Check sheet for the drawn part. Datum: minimum x, y, z corner. Units: mm. A direction names the side the tool comes from. Round coordinates to 2 decimals unless told otherwise and drop trailing zeros. Write each loop counter-clockwise with the first axis right and the second up, starting at its lowest first coordinate (ties: lowest second). Pieces come first, ordered by that corner, then holes. Notation, with made-up numbers: M 11,69.5 L 39,69.5 A17 ccw 39,97.5 Z; hole C 47,35 d11. An arc over 180 degrees is marked long. Put each result on its own line as item: value.
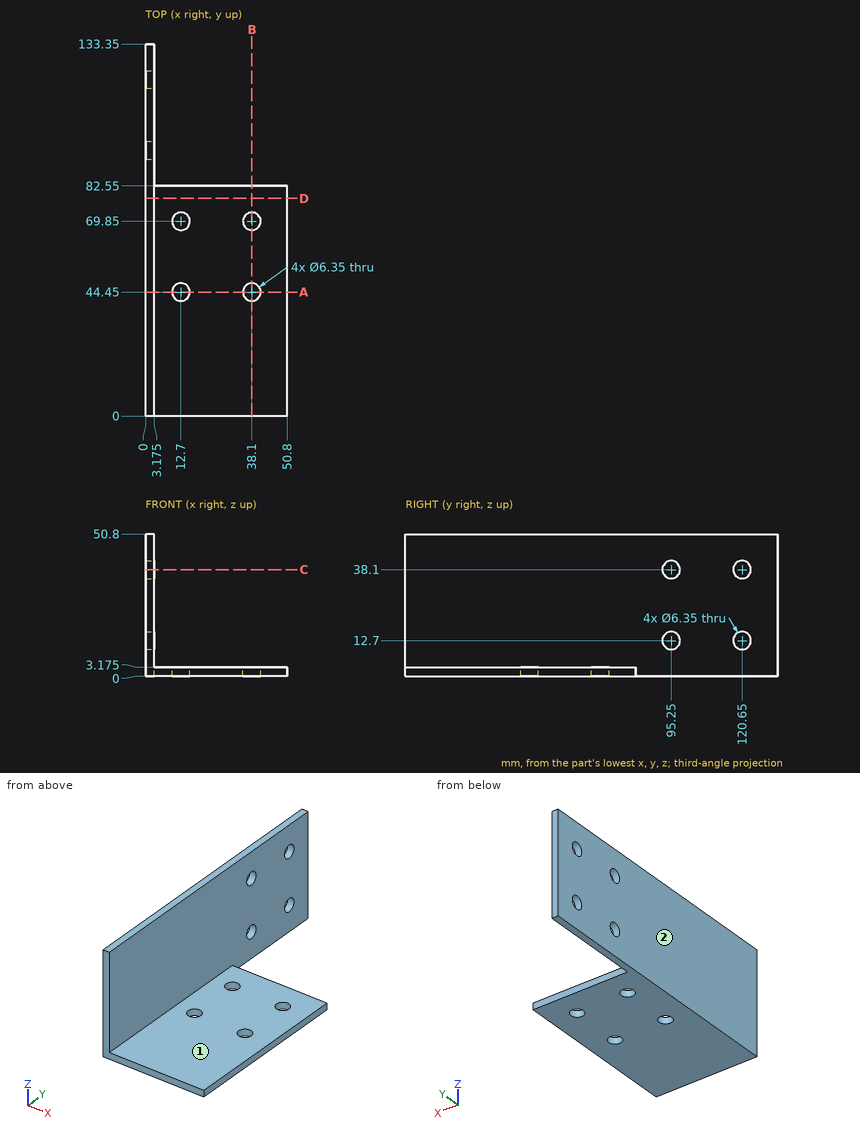
1. Cross-section at B-B (x = 38.1). Enter the section's corners in (y, z) (3 decimals), then the cut area to 3 significant figures.
Computed values:
outline: M 0,0 L 41.275,0 L 41.275,3.175 L 0,3.175 Z; M 47.625,0 L 66.675,0 L 66.675,3.175 L 47.625,3.175 Z; M 73.025,0 L 82.55,0 L 82.55,3.175 L 73.025,3.175 Z
area: 222 mm2
2. Scan lines: probe 1 along X at (y, z) = (44.45, 1.9) (3 decimals); probe 2 along Y at (x, z) = (2, 38); probe 3 along Y at (x, z) = (12.7, 1.5) (3 decimals). Record each from-to range of solid material in increasing order.
Computed values:
probe 1: x = 0 to 9.525, 15.875 to 34.925, 41.275 to 50.8
probe 2: y = 0 to 92.08, 98.42 to 117.48, 123.82 to 133.35
probe 3: y = 0 to 41.275, 47.625 to 66.675, 73.025 to 82.55
3. Access from +Z, -Z, +X, -X, +Y, -Y to the whole of each face (thin tool, end or side, straight path). Record for the marked faces 1 and 2.
Computed values:
face 1: +Z, +X, +Y, -Y
face 2: +Z, -Z, -X, +Y, -Y
4. Cross-section at C-C (z = 38.1). Enter the section's corners in (x, y) (3 decimals).
Computed values:
outline: M 0,0 L 3.175,0 L 3.175,92.075 L 0,92.075 Z; M 0,98.425 L 3.175,98.425 L 3.175,117.475 L 0,117.475 Z; M 0,123.825 L 3.175,123.825 L 3.175,133.35 L 0,133.35 Z
5. Cross-section at A-A (y = 44.45). Enter the section's corners in (x, z) (3 decimals), then the cut area to 3 significant figures.
Computed values:
outline: M 0,0 L 9.525,0 L 9.525,3.175 L 3.175,3.175 L 3.175,50.8 L 0,50.8 Z; M 15.875,0 L 34.925,0 L 34.925,3.175 L 15.875,3.175 Z; M 41.275,0 L 50.8,0 L 50.8,3.175 L 41.275,3.175 Z
area: 272 mm2
6. Depth check by flat-ended pin: pin 1 Ø8.5 at (y, z) = (120.65, 12.7) entering from +X (3 decimals); pin 2 Ø5 at (x, y) = (38.1, 69.85) entering from +Z; pin 3 Ø24 at (x, y) = (28, 53) entering from +Z (3 decimals); pin 4 Ø2.5 at (x, z) = (34, 2.5) entering from +Y. Enter the tip coordinate at first touch or a pass-through.
Computed values:
pin 1: stops at x = 3.175
pin 2: passes through
pin 3: stops at z = 3.175
pin 4: stops at y = 82.55
7. Cross-section at D-D (y = 78). Enter the section's corners in (x, z) (3 decimals).
Computed values:
outline: M 0,0 L 50.8,0 L 50.8,3.175 L 3.175,3.175 L 3.175,50.8 L 0,50.8 Z
